Geometry: final body of the model. Coordinates: model frame, mm. A direction names the side the tool comes from. Coordinates: 2 decimals unless noted, no trailing zeros. Order: outer loops, then holes, each group sorted by start corner. A loop starts at its lowest first (then second) coordinate and runs counter-clockwise, first axis right, second up. Notation, with made-up numbers: (-6, 21) -> (52, 21) arc R22 ccw to (52, 33) -> close; hole circle Ø7 at (47, 18). An arc over 180 degrees is marked (long way). Answer in a Markdown table with one row per item. Add a question column.
1) Ray query, line 1 (Z direction, x = 16.5, y = 7); line 2 (X direction, y = -16, z = 3); line 3 (Y direction, x = -5, z = 18.5). Return the intervals inside material, ascending. Write a range as from..to.
2) Section query B-B on x = 0. Count the separate pieces of the cut face and the enclosed holes in it, then the cut area to 3 significant figures.
3) Contact query for flat-ended pins moving along their axis: P1, Ø12, axis at x = 1, z = 23, coming from the -Y side; P2, Ø8, axis at x = 1, y = 16.5, coming from the -Z side; P3, Ø6, axis at x = 16, y = 0, coming from the +Z side; P4, Ø2, axis at y = -0.5, z = 22, coming from the +X side. Output: stop coordinate, or through.
4) Set-up query: faces 5 (the face through (2, -6, 30)), 6 (the face through (14, -2, 4.1)), 7 (the face through (-9, 9, 6)). Return all of +Z, -Z, +X, -X, +Y, -Y with unobstructed straight access to the full face (end or side cutting, diameter ignored); none if empty.
5) Pull-direction query (Y, two-part tool) for faces 1 (the face through (2, 14, 4.1)), 2 (the face through (-2, -6, 0)), 3 (the face through (1.73, 7.81, 0.25)), 4 (the face through (-10, -3.2, 17.9)); classes: +Y half, -Y half, draft (parallel to the pull), parting line (faces both ways), or undercut.
6) Section query A-A on z = 3. Return the cut outline in (x, y).
7) Section query D-D on z = 9. Return the cut outline in (x, y), then the cut area to 3 significant figures.
```python
from build123d import *

# Parameters (mm, degrees)
PADR_OCIRCULAR1_COUNT = 4
FILETE1_R             = 0.5


with BuildPart() as part:
    # Esboço1 → Revolução1 (revolve)
    with BuildSketch(Plane(origin=(0, 0, 0), x_dir=(0, 0, -1), z_dir=(1, 0, 0)), mode=Mode.PRIVATE) as revolu_o1_sk:
        Polygon((0, 6), (0, 8), (-0.5, 8), (-0.5, 8.5), (0, 8.5), (0, 10), (-0.5, 10), (-0.5, 10.5), (0, 10.5), (0, 21), (-6, 21), (-6, 10.5), (-30, 10.5), (-30, 8.5), (-29.5, 8.5), (-29.5, 8), (-30, 8), (-30, 6), align=None)
    revolve(revolu_o1_sk.sketch.rotate(Axis((0, 0, 0), (0, 0, 1)), 90), axis=Axis((0, 0, 0), (0, 0, 1)))  # turned: the seam where the file's is

    # Esboço5 → Corte-Revolução1 (revolve, cut)
    with BuildSketch(Plane(origin=(0, 0, 0), x_dir=(0, 0, -1), z_dir=(1, 0, 0)), mode=Mode.PRIVATE) as corte_revolu_o1_sk:
        Polygon((0, 19.75), (-4.1, 19.75), (-4.1, 18.25), (-6, 18.25), (-6, 16), (0, 16), align=None)
    corte_revolu_o1 = revolve(corte_revolu_o1_sk.sketch.rotate(Axis((0, 16, 0), (0, 0, -1)), 180), axis=Axis((0, 16, 0), (0, 0, -1)), mode=Mode.SUBTRACT)  # turned: the seam where the file's is

    # PadrãoCircular1: Corte-Revolução1 ×4 about axis
    padr_ocircular1_axis = Axis((0, 0, 0), (0, 0, 1))
    for i in range(1, PADR_OCIRCULAR1_COUNT):
        add(corte_revolu_o1.rotate(padr_ocircular1_axis, i * 360 / PADR_OCIRCULAR1_COUNT), mode=Mode.SUBTRACT)

    # Filete1
    filete1_edges = [part.edges().sort_by_distance(p)[0] for p in [
        (10.5, 0, 30),
        (21, 0, 6),
        (21, 0, 0),
    ]]
    fillet(filete1_edges, radius=FILETE1_R)


solid = part.part
```
Result:
| question | item | result |
|---|---|---|
| 1 | line 1 | 0..6 |
| 1 | line 2 | -13.6..-3.75, 3.75..13.6 |
| 1 | line 3 | -9.23..-3.32, 3.32..9.23 |
| 2 | separate pieces | 4 |
| 2 | enclosed holes | 0 |
| 2 | area | 316 mm2 |
| 3 | P1 | y = -10.5 |
| 3 | P2 | z = 0 |
| 3 | P3 | z = 6 |
| 3 | P4 | x = 10.5 |
| 4 | face 5 | +Z, +X, -X, +Y, -Y |
| 4 | face 6 | -Z |
| 4 | face 7 | +Z |
| 5 | face 1 | undercut |
| 5 | face 2 | draft |
| 5 | face 3 | undercut |
| 5 | face 4 | parting line |
| 6 | outline | circle Ø42 at (0, 0); hole circle Ø7.5 at (-16, 0); hole circle Ø12 at (0, 0); hole circle Ø7.5 at (0, -16); hole circle Ø7.5 at (0, 16); hole circle Ø7.5 at (16, 0) |
| 7 | outline | circle Ø21 at (0, 0); hole circle Ø12 at (0, 0) |
| 7 | area | 233 mm2 |
